Design review of the part built by this model. Coordinates are the model's own, in mm. Face numbers are marked on the shaded views. A direction names the side the tool comes from. Round coordinates to 2 decimals unless told otherwise and drop trailing zeros. Write each loop counter-clockwise with the first axis right and the second up, starting at its lowest first coordinate (ties: lowest second). Pieces come first, ordered by that corner, then holes. Notation, with made-up numbers: (83, 65.25) -> (99, 65.25) arc R24 ccw to (99, 75.25) -> close; hole circle Ø4 at (73.25, -32.5). An arc over 180 degrees is marked (long way). Write item = value, one per line. Start each with the question number.
Item 1: To check wall thickness, follow L1, parallel to Y at x = 234, z = 16; L2, parallel to Z at x = 55, y = 87.5; L3, parallel to Y at x = 128, z = -31. State the ranges of each line that lie inside material, in increasing order.
Item 2: Add section C-C, the plane z = 5. State the section outline as (x, y) points, then the cut area to 3 significant figures.
Item 3: Add section A-A, the plane x = 30. State the section outline as (y, z) points, then the cut area to 3 significant figures.
Item 4: Add section D-D, the plane y = 99. State the section outline as (x, z) points.
Item 5: Machinability: for the marked faces 4, 5, 6, 7 and 8, which of the approach directions +Z, -Z, +X, -X, +Y, -Y give a long, thin tool a straight path to every point of the face, cutting with its end or side? Answer none if there is none.
Item 6: Add section B-B, the plane z = -43. State the section outline as (x, y) points, then the cut area to 3 significant figures.
Item 7: Mouldability with a two-part tool opening along Z and no side actions: class the marked faces 1, 2 and 3 as released by +Z, released by -Z, zero draft, split by the parting line, or undercut.
Item 8: For pin 1 Ø1 at (x, y) = (34, 32) entering from +Z; pin 2 Ø1 at (x, z) = (33, -13.5) entering from +Y; pin 3 Ø1 at (x, z) = (207.5, 8.5) entering from +Y; pin 4 Ø12 at (y, z) = (57.5, -36) entering from +X, all flat-tipped, find the tip position at first contact; note any pin that passes through.
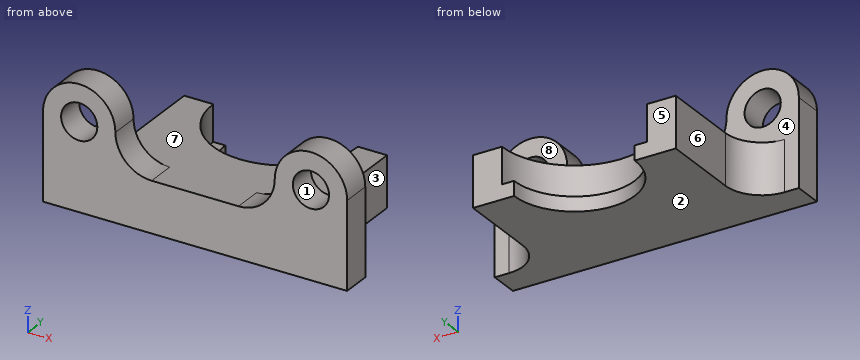
from build123d import *

# Parameters (mm, degrees)
SKETCH_1_R          = 15
EXTRUDE_1_DEPTH     = 24
SKETCH_3_W          = 168
SKETCH_3_H          = 96
EXTRUDE_2_DEPTH     = 42
SKETCH_4_R          = 60
CUT_EXTRUDE_1_DEPTH = 30
SKETCH_5_R          = 50
CUT_EXTRUDE_2_DEPTH = 30
FILLET_1_R          = 30


with BuildPart() as part:
    # 草圖1 → 填料-伸長1 (new body)
    # profile 1 of 2: a face of its own
    with BuildSketch(Plane(origin=(0, 0, 0), x_dir=(1, 0, 0), z_dir=(0, 1, 0))):
        with BuildLine():
            Line((252, 72), (126, 72))
            Line((126, 72), (126, 30))
            Line((126, 30), (162, 30))
            ThreePointArc((162, 30), (183.213203436, 21.213203436), (192, 0))
            ThreePointArc((192, 0), (222, -30), (252, 0))
            Line((252, 0), (252, 72))
        make_face()
        with Locations(Location((222, 0, 0), (0, 0, 270))):
            Circle(SKETCH_1_R, mode=Mode.SUBTRACT)
    # profile 2 of 2: a face of its own
    with BuildSketch(Plane(origin=(0, 0, 0), x_dir=(1, 0, 0), z_dir=(0, 1, 0))):
        with BuildLine():
            Line((0, 72), (0, 0))
            ThreePointArc((0, 0), (30, -30), (60, 0))
            ThreePointArc((60, 0), (68.786796564, 21.213203436), (90, 30))
            Line((90, 30), (126, 30))
            Line((126, 30), (126, 72))
            Line((126, 72), (0, 72))
        make_face()
        with Locations(Location((30, 0, 0), (0, 0, 270))):
            Circle(SKETCH_1_R, mode=Mode.SUBTRACT)
    extrude(amount=EXTRUDE_1_DEPTH)

    # 草圖3 → 填料-伸長2 (add)
    with BuildSketch(Plane(origin=(0, 0, -72), x_dir=(-1, 0, 0), z_dir=(0, 0, -1))):
        with Locations((-126, 72)):
            Rectangle(SKETCH_3_W, SKETCH_3_H)
    extrude(amount=-EXTRUDE_2_DEPTH)

    # 草圖4 → 除料-伸長1 (cut)
    with BuildSketch(Plane.XY.offset(-30)):
        with Locations((126, 120)):
            Circle(SKETCH_4_R)
    extrude(amount=-CUT_EXTRUDE_1_DEPTH, mode=Mode.SUBTRACT)

    # 草圖5 → 除料-伸長2 (cut)
    with BuildSketch(Plane.XY.offset(-60)):
        with Locations((126, 120)):
            Circle(SKETCH_5_R)
    extrude(amount=-CUT_EXTRUDE_2_DEPTH, mode=Mode.SUBTRACT)

    # 圓角1
    fillet_1_edges = [part.edges().sort_by_distance(p)[0] for p in [
        (42, 24, -51),
        (210, 24, -51),
    ]]
    fillet(fillet_1_edges, radius=FILLET_1_R)


solid = part.part
Result set:
q1.L1 = 0 to 24
q1.L2 = -72 to -30
q1.L3 = 0 to 60.03
q2.outline = (0.42, 0) -> (15.86, 0) -> (15.86, 24) -> (0.42, 24) -> close; (44.14, 0) -> (59.58, 0) -> (59.58, 24) -> (44.14, 24) -> close; (192.42, 0) -> (207.86, 0) -> (207.86, 24) -> (192.42, 24) -> close; (236.14, 0) -> (251.58, 0) -> (251.58, 24) -> (236.14, 24) -> close
q2.area = 1,480 mm²
q3.outline = (0, -72) -> (30, -72) -> (30, -30) -> (24, -30) -> (24, -15) -> (0, -15) -> close; (0, 15) -> (24, 15) -> (24, 30) -> (0, 30) -> close
q3.area = 1,980 mm²
q4.outline = (42, -72) -> (80.62, -72) -> (80.62, -60) -> (69.8, -60) -> (69.8, -30) -> (42, -30) -> close; (171.38, -72) -> (210, -72) -> (210, -30) -> (182.2, -30) -> (182.2, -60) -> (171.38, -60) -> close
q5.face_4 = +Z, -X, +Y
q5.face_5 = +Z, -Z, +X, -X, +Y
q5.face_6 = +Z, -Z, -X, +Y
q5.face_7 = +Z, +Y
q5.face_8 = +Z, +X, +Y
q6.outline = (0, 0) -> (252, 0) -> (252, 24) -> (240, 24) arc R30 cw to (210, 54) -> (210, 120) -> (186, 120) arc R60 cw to (66, 120) -> (42, 120) -> (42, 54) arc R30 cw to (12, 24) -> (0, 24) -> close
q6.area = 16,900 mm²
q7.face_1 = undercut
q7.face_2 = released by -Z
q7.face_3 = zero draft
q8.pin_1 = -30
q8.pin_2 = through
q8.pin_3 = 24
q8.pin_4 = 210.1
